Can you work these out from the model? Positions are in its coordinate system, mm. Round coordinates to 2 decimals unless told otherwise and drop trailing zeros. Loops run counter-clockwise (first coordinate to the right, second up) from the corner with the lowest first, then second, coordinate; pieces in that order, holes last.
```python
from build123d import *

# Parameters (mm, degrees)
F1_DEPTH = 2.0955
F2_R     = 0.635
F3_DEPTH = 25.4
F4_W     = 1.5875
F4_H     = 2.5404572
F4_R     = 0.635
F5_DEPTH = 0.635


# Not quite as in the source:
# - a feature names something its author has since deleted; it is built from what else it names


with BuildPart() as f1:
    # F0 (on Right) → F1 (new body)
    with BuildSketch(Plane.YZ):
        with BuildLine():
            Line((51.3955118105, -18.3105177657), (51.3955118105, -19.5805177657))
            Line((51.3955118105, -19.5805177657), (53.9359690105, -19.5805177657))
            ThreePointArc((53.9359690105, -19.5805177657), (58.0135640106, -25.4388820379), (65.0510564446, -26.6309026629))
            Line((65.0510564446, -26.6309026629), (64.8478195071, -25.8786771446))
            ThreePointArc((64.8478195071, -25.8786771446), (57.9021718289, -24.2424946681), (53.9359690105, -18.3105177657))
            Line((53.9359690105, -18.3105177657), (51.3955118105, -18.3105177657))
        make_face()
    extrude(amount=F1_DEPTH)

    # F2 (on face) → F3 (cut)
    with BuildSketch(Plane(origin=(0, 0, -19.5805177657), x_dir=(1, 0, 0), z_dir=(0, 0, -1))):
        with Locations((1.04775, -52.6657345776)):
            Circle(F2_R)
    extrude(amount=-F3_DEPTH, mode=Mode.SUBTRACT)

    # F4 (on face) → F5 (cut)
    with BuildSketch(Plane.XY.offset(-18.3105177657)):
        with Locations((1.04775, 52.6657404105)):
            Rectangle(F4_W, F4_H)
        with Locations((1.04775, 52.6657345776)):
            Circle(F4_R, mode=Mode.SUBTRACT)
    extrude(amount=-F5_DEPTH, mode=Mode.SUBTRACT)


solid = f1.part
```
(1) For pin 1 (0.6 mm diameter, centred on x = 1.5, y = 53, fed in from -Z); pin 2 (0.5 mm diameter, centred on x = 1, z = -18.5, fed in from -Y); pin 3 (1 mm diameter, centred on x = 1.5, z = -21.5, fed in from +Y), each with a flat end and sliding along its axis, tell me the tip position at first contact or that it passes through.
(2) Suppose I cut it at A-A (x = 1.05). Write out the boundary of the cut face in (y, z), then the cut area to 3 significant figures.
(3) Suppose I cut it at B-B (y = 58.75). Write out the boundary of the cut face in (x, z).
(4) Suppose I cut it at C-C (z = -26.25). Write out the boundary of the cut face in (x, y).
(5) We'd pull the mould along Y, two halves only. Please class faces 1 (the flat face through (1, 51.396, -19.2)), 2 (the flat face through (0, 57, -24)), 3 (the cylindrical face through (0.91, 53.286, -19.267)), 4 (the cylindrical face through (1.033, 57.987, -24.3)): released by +Y, released by -Y, zero draft, split by the parting line, or undercut.
(6) If I drill on line 1 (Z direction, x = 0.45, y = 56); line 2 (Y direction, x = 1.5, z = -20.75); line 3 (Z direction, x = 0.5, y = 59), over which ranges is the centre line in solid material (lowest first)?
Check result:
1. pin 1: stops at z = -19.58
1. pin 2: stops at y = 53.94
1. pin 3: stops at y = 55.6
2. outline: (51.4, -19.58) - (52.03, -19.58) - (52.03, -18.95) - (51.4, -18.95) - close; (53.3, -19.58) - (53.94, -19.58) arc R9.22 ccw to (65.05, -26.63) - (64.85, -25.88) arc R9.74 cw to (53.94, -18.31) - (53.94, -18.95) - (53.3, -18.95) - close
2. area: 12.4 mm2
3. outline: (0, -25.86) - (2.1, -25.86) - (2.1, -24.77) - (0, -24.77) - close
4. outline: (0, 59.62) - (2.1, 59.62) - (2.1, 64.95) - (0, 64.95) - close
5. face 1: released by -Y
5. face 2: zero draft
5. face 3: undercut
5. face 4: undercut
6. line 1: z = -23.71 to -22.51
6. line 2: y = 54.27 to 54.82
6. line 3: z = -25.98 to -24.9
